from build123d import *

# Parameters (mm, degrees)
SKETCH1_R           = 2
BOSS_EXTRUDE1_DEPTH = 30
SKETCH2_W           = 24
SKETCH2_H           = 19.394542589
CUT_EXTRUDE1_DEPTH  = 43.435404183
SKETCH3_R           = 8.9
SKETCH3_R_2         = 2
CUT_EXTRUDE2_DEPTH  = 3


with BuildPart() as part:
    # Sketch1 → Boss-Extrude1 (new body)
    with BuildSketch(Plane.XY):
        with BuildLine():
            Line((-10, 22.377746272), (0, 22.377746272))
            Line((0, 22.377746272), (10, 4.672746272))
            Line((10, 4.672746272), (10, -13.032253728))
            ThreePointArc((10, -13.032253728), (0, -16.426796317), (-10, -13.032253728))
            Line((-10, -13.032253728), (-10, 22.377746272))
        make_face()
        with Locations((0, -7.032253728)):
            Circle(SKETCH1_R, mode=Mode.SUBTRACT)
        with Locations((6, -7.032253728)):
            Circle(SKETCH1_R, mode=Mode.SUBTRACT)
        with Locations((-6, -7.032253728)):
            Circle(SKETCH1_R, mode=Mode.SUBTRACT)
    extrude(amount=BOSS_EXTRUDE1_DEPTH)

    # Sketch2 → Cut-Extrude1 (cut, through all)
    with BuildSketch(Plane(origin=(10, 0, 0), x_dir=(0, 0, -1), z_dir=(1, 0, 0))):
        with Locations((-15, -6.729525023)):
            Rectangle(SKETCH2_W, SKETCH2_H)
    extrude(amount=-CUT_EXTRUDE1_DEPTH, mode=Mode.SUBTRACT)

    # Sketch3 → Cut-Extrude2 (cut)
    with BuildSketch(Plane.ZY.offset(10)):
        with Locations((15, 12.967746272)):
            Circle(SKETCH3_R)
        with Locations((15, 18.967746272)):
            Circle(SKETCH3_R_2, mode=Mode.SUBTRACT)
        with Locations((15, 6.967746272)):
            Circle(SKETCH3_R_2, mode=Mode.SUBTRACT)
        with Locations((9, 12.967746272)):
            Circle(SKETCH3_R_2, mode=Mode.SUBTRACT)
        with Locations((21, 12.967746272)):
            Circle(SKETCH3_R_2, mode=Mode.SUBTRACT)
    extrude(amount=-CUT_EXTRUDE2_DEPTH, mode=Mode.SUBTRACT)


solid = part.part
Here's how the part is built. I have some questions about the finished solid (model axes, mm). A direction names the side the tool comes from. Coordinates: 2 decimals unless noted, no trailing zeros. Order: outer loops, then holes, each group sorted by start corner. A loop starts at its lowest first (then second) coordinate and runs counter-clockwise, first axis right, second up. Notation, with made-up numbers: M 54.25,33.5 L 92.25,33.5 A16 ccw 92.25,40.5 Z; hole C 86,-12 d11. An arc over 180 degrees is marked long. Answer as CSV lines item,"result". Start each with the question number.
1. For pin 1 (5 mm diameter, centred on x = 4.5, y = 10.5, fed in from -Z); pin 2 (8 mm diameter, centred on x = 8, z = 8, fed in from +Y); pin 3 (3 mm diameter, centred on x = 4.5, z = 6.5, fed in from -Y); pin 4 (3.5 mm diameter, centred on x = 0, y = -7.03, fed in from -Z), each with a flat end and sliding along its axis, tell me the tip position at first contact or that it passes through.
2. I need wall thicknesses on line 1 (Z direction, x = 2.5, y = -13.5); line 2 (Y direction, x = -6.5, z = 26.75); line 3 (Y direction, x = 6, z = 1.85). Which ranges of each line are inside material? Lowest first, please. Write a range as [from, to].
3. On a 3-axis mill with a long thin cutter (end or side, diameter ignored), from which of +Z, -Z, +X, -X, +Y, -Y can I reach the whole of each face in a straight line? I mean faces 5 (the flat face through (-10, 13, 9)), 6 (the cylindrical face through (-8.521, 20.319, 13.526)), 7 (the flat face through (0.1, -4.7, 3)). Say none if no direction works.
4. I want a section at B-B, the plane z = 15. Write out the boundary of the cut face in (x, y), and give its area (3 significant figures).
5. I want a section at A-A, the plane x = -6. Write out the boundary of the cut face in (y, z).
6. I want a section at C-C, the plane y = 12.5. Write out the boundary of the cut face in (x, z), and give its area (3 significant figures).
7. I want a section at D-D, the plane x = 0.5. Write out the boundary of the cut face in (y, z), and give its area (3 significant figures).
8. We'd pull the mould along X, two halves only. Please class faces 1 (the cylindrical face through (-0.26, -5.05, 28.48)), 2 (the flat face through (4.93, 13.65, 14.79)), 3 (the cylindrical face through (-8, -7, 28)), 4 (the cylindrical face through (-8.521, 14.319, 7.526)): released by +X, released by -X, zero draft, split by the parting line, or undercut.
Recorded:
1,pin 1,"stops at z = 0"
1,pin 2,"stops at y = 15.3"
1,pin 3,"stops at y = 2.97"
1,pin 4,"passes through"
2,line 1,"z = [0, 3], [27, 30]"
2,line 2,"y = [2.97, 22.38]"
2,line 3,"y = [-15.29, -9.03], [-5.03, 11.75]"
3,face 5,"+Z, -Z, -X, +Y, -Y"
3,face 6,"-X"
3,face 7,"+X, -X, -Y"
4,outline,"M -10,2.97 L 10,2.97 L 10,4.67 L 0,22.38 L -10,22.38 L -10,21.87 L -7,21.87 L -7,20.97 L -10,20.97 L -10,16.97 L -7,16.97 L -7,8.97 L -10,8.97 L -10,4.97 L -7,4.97 L -7,4.07 L -10,4.07 Z"
4,area,"270 mm2"
5,outline,"M -15.29,0 L -9.03,0 L -9.03,3 L -15.29,3 Z; M -15.29,27 L -9.03,27 L -9.03,30 L -15.29,30 Z; M -5.03,0 L 22.38,0 L 22.38,30 L -5.03,30 L -5.03,27 L 2.97,27 L 2.97,3 L -5.03,3 Z"
6,outline,"M -10,0 L 5.58,0 L 5.58,30 L -10,30 L -10,23.89 L -7,23.89 L -7,22.94 L -10,22.94 L -10,19.06 L -7,19.06 L -7,10.94 L -10,10.94 L -10,7.06 L -7,7.06 L -7,6.11 L -10,6.11 Z"
6,area,"437 mm2"
7,outline,"M -16.42,0 L -8.97,0 L -8.97,3 L -16.42,3 Z; M -16.42,27 L -8.97,27 L -8.97,30 L -16.42,30 Z; M -5.1,0 L 21.49,0 L 21.49,30 L -5.1,30 L -5.1,27 L 2.97,27 L 2.97,3 L -5.1,3 Z"
7,area,"649 mm2"
8,face 1,"undercut"
8,face 2,"released by +X"
8,face 3,"undercut"
8,face 4,"zero draft"
